Build history of the part. All positions in model axes, mm. A direction names the side the tool comes from. Round coordinates to 2 decimals unless told otherwise and drop trailing zeros. Loops run counter-clockwise (first coordinate to the right, second up) from the corner with the lowest first, then second, coordinate; pieces in that order, holes last. Notation, with made-up numbers: (54.25, 16.5) -> (86.25, 16.5) arc R18 ccw to (86.25, 41.5) -> close; hole circle Ø8 at (-29, 14). An arc over 180 degrees is marked (long way). Put each result on its own line as item: value. Start each with the question number.
Item 1: Cut at C-C, the plane y = -3.25. List the corners of the cut face in (x, z), plus the area to 3 significant figures.
Item 2: Flat gauge pins, fed straight in: pin 1 Ø12 at (x, z) = (1, 29.5) entering from -Y; pin 2 Ø2 at (y, z) = (7.5, 22.5) entering from +X; pin 3 Ø4 at (x, y) = (8.5, 0.5) entering from +Z. Where does each tip first touch, or does it go through?
Item 3: Cut at B-B, the plane z = 51. List the corners of the cut face in (x, y).
Item 4: Drill centre lines: probe 1 along Z at (x, y) = (5.75, 0); probe 2 along Z at (x, y) = (-9, 5); probe 3 along Z at (x, y) = (-7.25, -0.75). Where is each one in solid material? Low to high. Write a range as [from, to].
Item 5: Pull direction X, two halves, no side cores. Call faces 1 (the cylindrical face through (-8.8, -0.6, 1.2)), 2 (the cylindrical face through (-6, -8, 35)), 3 (the flat face through (0, 0, 0)): +X half, -X half, draft (parallel to the pull), parting line (faces both ways), or undercut.
Item 6: Tool access for faces 4 (the cylindrical face through (5.68, 4.54, 35.21)), 5 (the cylindrical face through (0.81, 9.55, 3.77)), 6 (the flat face through (4, -6, 50)): list every direction of +Z, -Z, +X, -X, +Y, -Y with a clear straight run to the whole face (end or side of a thin tool).
Item 7: Cut at A-A, the plane y = 0. Count the separate pieces of the cut face and the enclosed holes in it, plus the area to 3 significant figures.
```python
from build123d import *

# Parameters (mm, degrees)
ESQUISSE1_R                        = 11
BOSS_EXTRU_1_DEPTH                 = 5
ENL_V_MAT_EXTRU_1_DEPTH            = 17.340134638
ESQUISSE3_R                        = 5
BOSS_EXTRU_2_DEPTH                 = 57.75
BOSS_EXTRU_3_DEPTH                 = 15
CONG_1_R                           = 1
R_P_TITION_CIRCULAIRE1_COUNT       = 5
CONG_1_OF_R_P_TITION_CIRCULAIRE1_R = 1
ESQUISSE3D1_R                      = 1.75
ENL_V_MAT_EXTRU_2_DEPTH            = 2.5
ENL_V_MAT_EXTRU_3_OUTLINE_R        = 1
ENL_V_MAT_EXTRU_3_DEPTH            = 2.5


# Read off the part's stored shape, not the designer's step: Enlèv. mat.-Extru.3
with BuildPart() as part:
    # Esquisse1 → Boss.-Extru.1 (new body)
    with BuildSketch(Plane.XY):
        Circle(ESQUISSE1_R)
    extrude(amount=BOSS_EXTRU_1_DEPTH)

    # Esquisse2 → Enlèv. mat.-Extru.1 (cut, through all)
    with BuildSketch(Plane.XY.offset(5)):
        with BuildLine():
            ThreePointArc((1, 8), (0.707106781, 8.707106781), (0, 9))
            Line((0, 9), (0, 8))
            ThreePointArc((0, 8), (0.5, 7.984359711), (0.998044964, 7.9375))
            ThreePointArc((0.998044964, 7.9375), (0.999511121, 7.968734715), (1, 8))
        make_face()
        with BuildLine():
            Line((0, 8), (0, 9))
            ThreePointArc((0, 9), (-0.728868987, 8.684653197), (-0.998044964, 7.9375))
            ThreePointArc((-0.998044964, 7.9375), (-0.5, 7.984359711), (0, 8))
        make_face()
        with BuildLine():
            ThreePointArc((0.998044964, 7.9375), (0.5, 7.984359711), (0, 8))
            Line((0, 8), (0, 7))
            ThreePointArc((0, 7), (0.684653197, 7.271131013), (0.998044964, 7.9375))
        make_face()
        with BuildLine():
            Line((0, 7), (0, 8))
            ThreePointArc((0, 8), (-0.5, 7.984359711), (-0.998044964, 7.9375))
            ThreePointArc((-0.998044964, 7.9375), (-0.684653197, 7.271131013), (0, 7))
        make_face()
        with BuildLine():
            ThreePointArc((0, -7), (-0.684653197, -7.271131013), (-0.998044964, -7.9375))
            ThreePointArc((-0.998044964, -7.9375), (-0.5, -7.984359711), (0, -8))
            Line((0, -8), (0, -7))
        make_face()
        with BuildLine():
            ThreePointArc((0, -8), (-0.5, -7.984359711), (-0.998044964, -7.9375))
            ThreePointArc((-0.998044964, -7.9375), (-0.728868987, -8.684653197), (0, -9))
            Line((0, -9), (0, -8))
        make_face()
        with BuildLine():
            ThreePointArc((0.998044964, -7.9375), (0.684653197, -7.271131013), (0, -7))
            Line((0, -7), (0, -8))
            ThreePointArc((0, -8), (0.5, -7.984359711), (0.998044964, -7.9375))
        make_face()
        with BuildLine():
            ThreePointArc((0.998044964, -7.9375), (0.5, -7.984359711), (0, -8))
            Line((0, -8), (0, -9))
            ThreePointArc((0, -9), (0.707106781, -8.707106781), (1, -8))
            ThreePointArc((1, -8), (0.999511121, -7.968734715), (0.998044964, -7.9375))
        make_face()
    extrude(amount=-ENL_V_MAT_EXTRU_1_DEPTH, mode=Mode.SUBTRACT)

    # Esquisse3 → Boss.-Extru.2 (add)
    with BuildSketch(Plane.XY.offset(5)):
        Circle(ESQUISSE3_R)
    extrude(amount=BOSS_EXTRU_2_DEPTH)

    # Esquisse4 → Boss.-Extru.3 (add, symmetric)
    with BuildSketch(Plane.XY.offset(35)):
        with BuildLine():
            ThreePointArc((-2.731158071, 4.188170912), (-2.5, 7.120566641), (-1.5, 9.886859967))
            ThreePointArc((-1.5, 9.886859967), (0, 10), (1.5, 9.886859967))
            ThreePointArc((1.5, 9.886859967), (2.5, 7.120566641), (2.731158071, 4.188170912))
            ThreePointArc((2.731158071, 4.188170912), (0, -5), (-2.731158071, 4.188170912))
        make_face()
    boss_extru_3 = extrude(amount=BOSS_EXTRU_3_DEPTH, both=True)

    # Congé1
    cong_1_edges = [part.edges().sort_by_distance(p)[0] for p in [
        (1.5, 9.886859967, 35),
        (-1.5, 9.886859967, 35),
    ]]
    fillet(cong_1_edges, radius=CONG_1_R)

    # Répétition circulaire1: Boss.-Extru.3 ×5 about axis
    r_p_tition_circulaire1_axis = Axis((0, 0, 0), (0, 0, 1))
    for i in range(1, R_P_TITION_CIRCULAIRE1_COUNT):
        add(boss_extru_3.rotate(r_p_tition_circulaire1_axis, i * 360 / R_P_TITION_CIRCULAIRE1_COUNT))

    # Congé1 of Répétition circulaire1
    cong_1_of_r_p_tition_circulaire1_edges = [part.edges().sort_by_distance(p)[0] for p in [
        (-8.939437105, 4.481792525, 35),
        (-9.866488089, 1.628622976, 35),
        (-7.024875971, -7.116959856, 35),
        (-4.597824988, -8.880315612, 35),
        (4.597824988, -8.880315612, 35),
        (7.024875971, -7.116959856, 35),
        (9.866488089, 1.628622976, 35),
        (8.939437105, 4.481792525, 35),
    ]]
    fillet(cong_1_of_r_p_tition_circulaire1_edges, radius=CONG_1_OF_R_P_TITION_CIRCULAIRE1_R)

    # Esquisse3D1 → Enlèv. mat.-Extru.2 (cut)
    with BuildSketch(Plane(origin=(0, -8, 5), x_dir=(0, 1, 0), z_dir=(-7.673874556635152e-12, 0, -1.0))):
        with Locations(Location((0, 0, 0), (0, 0, 90))):
            Circle(ESQUISSE3D1_R)
        with Locations(Location((8, 8, 0), (0, 0, 270))):
            Circle(ESQUISSE3D1_R)
        with Locations(Location((8, -8, 0), (0, 0, 270))):
            Circle(ESQUISSE3D1_R)
        with Locations(Location((16, 0, 0), (0, 0, 90))):
            Circle(ESQUISSE3D1_R)
    extrude(amount=ENL_V_MAT_EXTRU_2_DEPTH, mode=Mode.SUBTRACT)

    # Enlèv. mat.-Extru.3 outline → Enlèv. mat.-Extru.3 (cut)
    with BuildSketch(Plane.XY):
        with Locations((8, 0)):
            Circle(ENL_V_MAT_EXTRU_3_OUTLINE_R)
        with Locations((-8, 0)):
            Circle(ENL_V_MAT_EXTRU_3_OUTLINE_R)
    extrude(amount=ENL_V_MAT_EXTRU_3_DEPTH, mode=Mode.SUBTRACT)


solid = part.part
```
Reply:
1. outline: (-10.51, 0) -> (10.51, 0) -> (10.51, 5) -> (3.8, 5) -> (3.8, 20) -> (5.68, 20) -> (5.68, 50) -> (3.8, 50) -> (3.8, 62.75) -> (-3.8, 62.75) -> (-3.8, 50) -> (-5.68, 50) -> (-5.68, 20) -> (-3.8, 20) -> (-3.8, 5) -> (-10.51, 5) -> close
1. area: 657 mm^2
2. pin 1: stops at y = -8.74
2. pin 2: stops at x = 2.62
2. pin 3: stops at z = 50
3. outline: circle Ø10 at (0, 0)
4. probe 1: z = [0, 5], [20, 50]
4. probe 2: z = [0, 5]
4. probe 3: z = [0, 2.5]
5. face 1: undercut
5. face 2: -X half
5. face 3: draft
6. face 4: +Z, +Y
6. face 5: none
6. face 6: +Z, +X, -Y
7. separate pieces: 3
7. enclosed holes: 0
7. area: 830 mm^2
